```python
from build123d import *

# Parameters (mm, degrees)
F0_W     = 16.768251
F0_H     = 110
F0_W_2   = 16.76825
F1_DEPTH = 3


# Not quite as in the source:
# - ends of sketch curves that miss each other by under 0.0002 mm in the source are joined


with BuildPart() as f1:
    # F0 (on Front) → F1 (new body)
    with BuildSketch(Plane.XZ):
        with BuildLine():
            Line((-165.473004, -55), (-165.473004, 55))
            Line((-165.473004, 55), (-168.473004, 55))
            Line((-168.473004, 55), (-168.473004, 52))
            Line((-168.473004, 52), (-180.473004, 52))
            Line((-180.473004, 52), (-180.473004, 55))
            Line((-180.473004, 55), (-188.473004, 55))
            Line((-188.473004, 55), (-188.473004, 52))
            Line((-188.473004, 52), (-193.223004, 52))
            Line((-193.223004, 52), (-193.223004, 44.5))
            ThreePointArc((-193.223004, 44.5), (-192.6518622233, 43.1211417767), (-191.273004, 42.55))
            Line((-191.273004, 42.55), (-187.887382, 42.55))
            ThreePointArc((-187.887382, 42.55), (-186.9753529387, 42.7764272596), (-186.2751272015, 43.4031251371))
            ThreePointArc((-186.2751272015, 43.4031251371), (-175.223004, 40), (-186.2751273913, 36.5968747338))
            ThreePointArc((-186.2751273913, 36.5968747338), (-186.9753529387, 37.2235727404), (-187.887382, 37.45))
            Line((-187.887382, 37.45), (-191.273004, 37.45))
            ThreePointArc((-191.273004, 37.45), (-192.6518622233, 36.8788582233), (-193.223004, 35.5))
            Line((-193.223004, 35.5), (-193.223004, 19.5))
            ThreePointArc((-193.223004, 19.5), (-192.6518622233, 18.1211417767), (-191.273004, 17.55))
            Line((-191.273004, 17.55), (-187.887382, 17.55))
            ThreePointArc((-187.887382, 17.55), (-186.9753529387, 17.7764272596), (-186.2751272015, 18.4031251371))
            ThreePointArc((-186.2751272015, 18.4031251371), (-175.223004, 15), (-186.2751273913, 11.5968747338))
            ThreePointArc((-186.2751273913, 11.5968747338), (-186.9753529387, 12.2235727404), (-187.887382, 12.45))
            Line((-187.887382, 12.45), (-191.273004, 12.45))
            ThreePointArc((-191.273004, 12.45), (-192.6518622233, 11.8788582233), (-193.223004, 10.5))
            Line((-193.223004, 10.5), (-193.223004, -10.5))
            ThreePointArc((-193.223004, -10.5), (-192.6518622233, -11.8788582233), (-191.273004, -12.45))
            Line((-191.273004, -12.45), (-187.887382, -12.45))
            ThreePointArc((-187.887382, -12.45), (-186.9753529387, -12.2235727404), (-186.2751272015, -11.5968748629))
            ThreePointArc((-186.2751272015, -11.5968748629), (-175.223004, -15), (-186.2751273913, -18.4031252662))
            ThreePointArc((-186.2751273913, -18.4031252662), (-186.9753529387, -17.7764272596), (-187.887382, -17.55))
            Line((-187.887382, -17.55), (-191.273004, -17.55))
            ThreePointArc((-191.273004, -17.55), (-192.6518622233, -18.1211417767), (-193.223004, -19.5))
            Line((-193.223004, -19.5), (-193.223004, -35.5))
            ThreePointArc((-193.223004, -35.5), (-192.6518622233, -36.8788582233), (-191.273004, -37.45))
            Line((-191.273004, -37.45), (-187.887382, -37.45))
            ThreePointArc((-187.887382, -37.45), (-186.9753529387, -37.2235727404), (-186.2751272015, -36.5968748629))
            ThreePointArc((-186.2751272015, -36.5968748629), (-175.223004, -40), (-186.2751273913, -43.4031252662))
            ThreePointArc((-186.2751273913, -43.4031252662), (-186.9753529387, -42.7764272596), (-187.887382, -42.55))
            Line((-187.887382, -42.55), (-191.273004, -42.55))
            ThreePointArc((-191.273004, -42.55), (-192.6518622233, -43.1211417767), (-193.223004, -44.5))
            Line((-193.223004, -44.5), (-193.223004, -55))
            Line((-193.223004, -55), (-180.473004, -55))
            Line((-180.473004, -55), (-180.473004, -52))
            Line((-180.473004, -52), (-168.473004, -52))
            Line((-168.473004, -52), (-168.473004, -55))
            Line((-168.473004, -55), (-165.473004, -55))
        make_face()
        with Locations((-157.0888785, 0)):
            Rectangle(F0_W, F0_H)
        with Locations((-140.3206275, 0)):
            Rectangle(F0_W, F0_H)
        Polygon((-58.336502, -55), (-58.336502, 55), (-64.336502, 55), (-64.336502, 52), (-84.336502, 52), (-84.336502, 55), (-105.936502, 55), (-105.936502, 52), (-125.936502, 52), (-125.936502, 55), (-131.936502, 55), (-131.936502, -55), (-125.936502, -55), (-125.936502, -52), (-105.936502, -52), (-105.936502, -55), (-84.336502, -55), (-84.336502, -52), (-64.336502, -52), (-64.336502, -55), align=None)
        with Locations((-33.1841255, 0)):
            Rectangle(F0_W, F0_H)
        Polygon((18.8, -55), (18.8, 55), (8, 55), (8, 52), (-14, 52), (-14, 55), (-24.8, 55), (-24.8, -55), (-14, -55), (-14, -52), (8, -52), (8, -55), align=None)
        with Locations((27.184125, 0)):
            Rectangle(F0_W_2, F0_H)
        with Locations((43.9523755, 0)):
            Rectangle(F0_W, F0_H)
        Polygon((125.936501, -55), (125.936501, 55), (119.936501, 55), (119.936501, 52), (99.936501, 52), (99.936501, 55), (78.336501, 55), (78.336501, 52), (58.336501, 52), (58.336501, 55), (52.336501, 55), (52.336501, -55), (58.336501, -55), (58.336501, -52), (78.336501, -52), (78.336501, -55), (99.936501, -55), (99.936501, -52), (119.936501, -52), (119.936501, -55), align=None)
        with Locations((134.3206265, 0)):
            Rectangle(F0_W, F0_H)
        with Locations((151.0888775, 0)):
            Rectangle(F0_W, F0_H)
        with BuildLine():
            Line((164.473003, 55), (159.473003, 55))
            Line((159.473003, 55), (159.473003, -55))
            Line((159.473003, -55), (175.223003, -55))
            Line((175.223003, -55), (175.223003, -44.5))
            ThreePointArc((175.223003, -44.5), (175.8234340986, -43.0504310986), (177.273003, -42.45))
            Line((177.273003, -42.45), (180.658624, -42.45))
            ThreePointArc((180.658624, -42.45), (181.6174238462, -42.6880389477), (182.3535586128, -43.3468752634))
            ThreePointArc((182.3535586128, -43.3468752634), (193.223003, -40), (182.3535591066, -36.6531250725))
            ThreePointArc((182.3535591066, -36.6531250725), (181.6174238462, -37.3119610523), (180.658624, -37.55))
            Line((180.658624, -37.55), (177.273003, -37.55))
            ThreePointArc((177.273003, -37.55), (175.8234340986, -36.9495689014), (175.223003, -35.5))
            Line((175.223003, -35.5), (175.223003, -19.5))
            ThreePointArc((175.223003, -19.5), (175.8234340986, -18.0504310986), (177.273003, -17.45))
            Line((177.273003, -17.45), (180.658624, -17.45))
            ThreePointArc((180.658624, -17.45), (181.6174238462, -17.6880389477), (182.3535586128, -18.3468752634))
            ThreePointArc((182.3535586128, -18.3468752634), (193.223003, -15), (182.3535591066, -11.6531250725))
            ThreePointArc((182.3535591066, -11.6531250725), (181.6174238462, -12.3119610523), (180.658624, -12.55))
            Line((180.658624, -12.55), (177.273003, -12.55))
            ThreePointArc((177.273003, -12.55), (175.8234340986, -11.9495689014), (175.223003, -10.5))
            Line((175.223003, -10.5), (175.223003, 10.5))
            ThreePointArc((175.223003, 10.5), (175.8234340986, 11.9495689014), (177.273003, 12.55))
            Line((177.273003, 12.55), (180.658624, 12.55))
            ThreePointArc((180.658624, 12.55), (181.6174238462, 12.3119610523), (182.3535586128, 11.6531247366))
            ThreePointArc((182.3535586128, 11.6531247366), (193.223003, 15), (182.3535591066, 18.3468749275))
            ThreePointArc((182.3535591066, 18.3468749275), (181.6174238462, 17.6880389477), (180.658624, 17.45))
            Line((180.658624, 17.45), (177.273003, 17.45))
            ThreePointArc((177.273003, 17.45), (175.8234340986, 18.0504310986), (175.223003, 19.5))
            Line((175.223003, 19.5), (175.223003, 35.5))
            ThreePointArc((175.223003, 35.5), (175.8234340986, 36.9495689014), (177.273003, 37.55))
            Line((177.273003, 37.55), (180.658624, 37.55))
            ThreePointArc((180.658624, 37.55), (181.6174238462, 37.3119610523), (182.3535586128, 36.6531247366))
            ThreePointArc((182.3535586128, 36.6531247366), (193.223003, 40), (182.3535591066, 43.3468749275))
            ThreePointArc((182.3535591066, 43.3468749275), (181.6174238462, 42.6880389477), (180.658624, 42.45))
            Line((180.658624, 42.45), (177.273003, 42.45))
            ThreePointArc((177.273003, 42.45), (175.8234340986, 43.0504310986), (175.223003, 44.5))
            Line((175.223003, 44.5), (175.223003, 52))
            Line((175.223003, 52), (164.473003, 52))
            Line((164.473003, 52), (164.473003, 55))
        make_face()
        with Locations((-49.9523765, 0)):
            Rectangle(F0_W, F0_H)
    extrude(amount=F1_DEPTH)


solid = f1.part
```
Source: CAD feature listing. Evaluate the final solid. Frame: model axes, mm. Coordinates: 2 decimals unless noted, no trailing zeros. Loops run counter-clockwise (first coordinate to the right, second up) from the corner with the lowest first, then second, coordinate; pieces in that order, holes last. Notation, with made-up numbers: M 82,-34.5 L 114,-34.5 A8 cw 114,-21.5 Z; hole C 29.5,54.5 d3. An arc over 180 degrees is marked long. Put each result on its own line as item: value. Start each with the question number.
1) Cut plane B-B on x = 113. Return the cut outline in (y, z).
2) Ray query, L1, parallel to X at y = -0.45, z = -36; L2, parallel to X at y = -2.9, z = -10.5; L3, parallel to X at y = -1.8, z = -5. Return the intervals inside material, ascending. Write a range as from..to.
3) Contact query for flat-ended pins moving along their axis: pin 1 Ø1.5 at (x, y) = (-191.5, -1.5) entering from +Z; pin 2 Ø0.9 at (y, z) = (-2, 53) entering from -X; pin 3 Ø0.9 at (y, z) = (-1.5, 53.5) entering from +X. Output: stop coordinate, or through.
4) Pull-direction query (X, two-part tool) for faces 1 (the face through (-175.227, -1.479, 40.215)), 2 (the face through (-3, -3, 1)); classes: pulls with the +X half, pulls with the -X half, needs draft (parallel to the pull), parting line crosses it, or undercut.
5) Cut plane A-A on z = 28. Return the cut outline in (x, y).
The answers:
1. outline: M -3,-52 L 0,-52 L 0,52 L -3,52 Z
2. L1: x = -193.16..-185.81, -176.73..175.28, 182.87..191.68
2. L2: x = -193.22..-185.32, -177.23..175.22, 183.38..191.17
2. L3: x = -193.22..175.22
3. pin 1: stops at z = 52
3. pin 2: stops at x = -188.47
3. pin 3: stops at x = 164.47
4. face 1: undercut
4. face 2: needs draft
5. outline: M -193.22,-3 L 175.22,-3 L 175.22,0 L -193.22,0 Z
